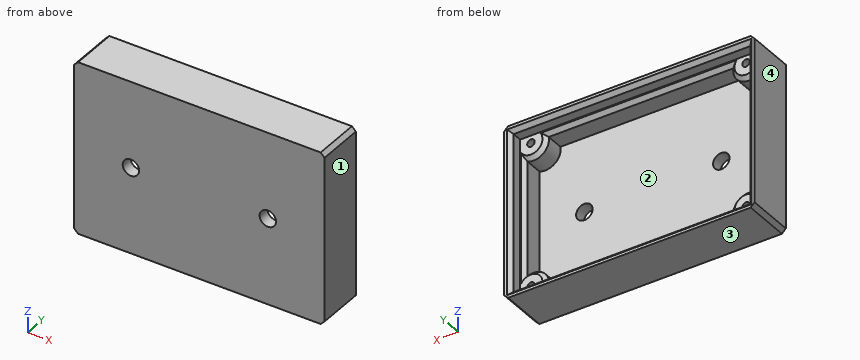
from build123d import *

# Parameters (mm, degrees)
SKETCH1_W           = 64
SKETCH1_H           = 44
BOSS_EXTRUDE1_DEPTH = 12
SKETCH2_W           = 60.5
SKETCH2_H           = 40.5
CUT_EXTRUDE1_DEPTH  = 3.5
SKETCH3_R           = 0.95
CUT_EXTRUDE2_DEPTH  = 6
SHELL1_START        = 3
SHELL1_DEPTH        = 5.5
CHAMFER1_SIZE       = 1
CHAMFER2_SIZE       = 1
CHAMFER3_SIZE       = 1
SKETCH4_R           = 2.1
CUT_EXTRUDE3_DEPTH  = 40.862262856


# Read off the part's stored shape, not the designer's step: Shell1
with BuildPart() as part:
    # Sketch1 → Boss-Extrude1 (new body)
    with BuildSketch(Plane(origin=(0, 0, 0), x_dir=(1, 0, 0), z_dir=(0, 1, 0))):
        Rectangle(SKETCH1_W, SKETCH1_H)
    extrude(amount=BOSS_EXTRUDE1_DEPTH)

    # Sketch2 → Cut-Extrude1 (cut)
    with BuildSketch(Plane(origin=(0, 12, 0), x_dir=(1, 0, 0), z_dir=(0, 1, 0))):
        Rectangle(SKETCH2_W, SKETCH2_H)
    extrude(amount=-CUT_EXTRUDE1_DEPTH, mode=Mode.SUBTRACT)

    # Sketch3 → Cut-Extrude2 (cut)
    with BuildSketch(Plane(origin=(0, 8.5, 0), x_dir=(1, 0, 0), z_dir=(0, 1, 0))):
        with Locations(Location((-27.5, 18.333333333, 0), (0, 0, 270))):
            Circle(SKETCH3_R)
        with Locations(Location((27.5, 18.333333333, 0), (0, 0, 270))):
            Circle(SKETCH3_R)
        with Locations(Location((27.5, -18.333333333, 0), (0, 0, 270))):
            Circle(SKETCH3_R)
        with Locations(Location((-27.5, -18.333333333, 0), (0, 0, 270))):
            Circle(SKETCH3_R)
    extrude(amount=-CUT_EXTRUDE2_DEPTH, mode=Mode.SUBTRACT)

    # Shell1 outline → Shell1 (cut)
    with BuildSketch(Plane(origin=(0, 0, 0), x_dir=(1, 0, 0), z_dir=(0, 1, 0)).offset(SHELL1_START)):
        with BuildLine():
            Line((-23.60666524, -19), (23.60666524, -19))
            ThreePointArc((23.60666524, -19), (25.030327008, -15.250604784), (29, -14.679226055))
            Line((29, -14.679226055), (29, 14.679226055))
            ThreePointArc((29, 14.679226055), (25.030327008, 15.250604784), (23.60666524, 19))
            Line((23.60666524, 19), (-23.60666524, 19))
            ThreePointArc((-23.60666524, 19), (-25.030327008, 15.250604784), (-29, 14.679226055))
            Line((-29, 14.679226055), (-29, -14.679226055))
            ThreePointArc((-29, -14.679226055), (-25.030327008, -15.250604784), (-23.60666524, -19))
        make_face()
    extrude(amount=SHELL1_DEPTH, mode=Mode.SUBTRACT)

    # Chamfer1
    chamfer1_edges = [part.edges().sort_by_distance(p)[0] for p in [
        (30.25, 12, 0),
        (0, 12, -20.25),
        (-30.25, 12, 0),
        (0, 12, 20.25),
    ]]
    chamfer(chamfer1_edges, length=CHAMFER1_SIZE)

    # Chamfer2
    chamfer2_edges = [part.edges().sort_by_distance(p)[0] for p in [
        (0, 8.5, 19),
        (29, 8.5, 0),
        (0, 8.5, -19),
        (-29, 8.5, 0),
        (-25.030327008, 8.5, -15.250604784),
        (25.030327008, 8.5, -15.250604784),
        (25.030327008, 8.5, 15.250604784),
        (-25.030327008, 8.5, 15.250604784),
    ]]
    chamfer(chamfer2_edges, length=CHAMFER2_SIZE)

    # Chamfer3
    chamfer3_edges = [part.edges().sort_by_distance(p)[0] for p in [
        (-32, 6, 22),
        (-32, 6, -22),
        (32, 6, -22),
        (32, 6, 22),
    ]]
    chamfer(chamfer3_edges, length=CHAMFER3_SIZE)

    # Sketch4 → Cut-Extrude3 (cut, through all)
    with BuildSketch(Plane(origin=(0, 3, 0), x_dir=(1, 0, 0), z_dir=(0, 1, 0))):
        with Locations(Location((-17.5, 0, 0), (0, 0, 270))):
            Circle(SKETCH4_R)
        with Locations(Location((17.5, 0, 0), (0, 0, 270))):
            Circle(SKETCH4_R)
    extrude(amount=-CUT_EXTRUDE3_DEPTH, mode=Mode.SUBTRACT)


solid = part.part
Here's how the part is built. I have some questions about the finished solid (model axes, mm). Face numbers are marked on the shaded views. Coordinates: 2 decimals unless noted, no trailing zeros. Order: outer loops, then holes, each group sorted by start corner. A loop starts at its lowest first (then second) coordinate and runs counter-clockwise, first axis right, second up. Notation, with made-up numbers: M -1.75,-19.75 L 30.25,-19.75 A10 cw 30.25,-14.75 Z; hole C 65,-11.75 d7. An arc over 180 degrees is marked long. Answer as CSV lines item,"result". Start each with the question number.
1. I want a section at D-D, the plane x = 27.5. Write out the boundary of the cut face in (y, z), and give its area (3 significant figures).
2. I want a section at B-B, the plane z = 0. Write out the boundary of the cut face in (x, y).
3. For pin 1 (1 mm diameter, centred on x = 25.5, z = 7, fed in from +Y); pin 2 (2 mm diameter, centred on x = -28, z = -18.5, fed in from +Y); pin 3 (0.6 mm diameter, centred on x = -27.5, z = 18.5, fed in from +Y), each with a flat end and sliding along its axis, tell me the tip position at first contact or that it passes through.
4. I want a section at A-A, the plane x = 17.5. Write out the boundary of the cut face in (y, z), and give its area (3 significant figures).
5. I want a section at C-C, the plane x = -13. Write out the boundary of the cut face in (y, z), and give its area (3 significant figures).
6. We'd pull the mould along X, two halves only. Please class the marked faces 1, 2, 3 and 4: released by +X, released by -X, zero draft, split by the parting line, or undercut.
7. I need wall thicknesses on line 1 (X direction, y = 1.9, z = 0); line 2 (Z direction, x = -3, y = 4.25); line 3 (Z direction, x = 21, y = 9.5). Which ranges of each line are inside material? Lowest first, please. Write a range as [from, to].
Recorded:
1,outline,"M 0,-22 L 12,-22 L 12,-21.25 L 11,-20.25 L 8.5,-20.25 L 8.5,-19.28 L 2.5,-19.28 L 2.5,-17.38 L 8.5,-17.38 L 8.5,-15.38 L 7.5,-14.38 L 3,-14.38 L 3,14.38 L 7.5,14.38 L 8.5,15.38 L 8.5,17.38 L 2.5,17.38 L 2.5,19.28 L 8.5,19.28 L 8.5,20.25 L 11,20.25 L 12,21.25 L 12,22 L 0,22 Z"
1,area,"203 mm2"
2,outline,"M -32,0 L -19.6,0 L -19.6,3 L -29,3 L -29,7.5 L -30,8.5 L -30.25,8.5 L -30.25,11 L -31.25,12 L -32,12 Z; M -15.4,0 L 15.4,0 L 15.4,3 L -15.4,3 Z; M 19.6,0 L 32,0 L 32,12 L 31.25,12 L 30.25,11 L 30.25,8.5 L 30,8.5 L 29,7.5 L 29,3 L 19.6,3 Z"
3,pin 1,"stops at y = 3"
3,pin 2,"stops at y = 8.5"
3,pin 3,"stops at y = 2.5"
4,outline,"M 0,-22 L 12,-22 L 12,-21.25 L 11,-20.25 L 8.5,-20.25 L 8.5,-20 L 7.5,-19 L 3,-19 L 3,-2.1 L 0,-2.1 Z; M 0,2.1 L 3,2.1 L 3,19 L 7.5,19 L 8.5,20 L 8.5,20.25 L 11,20.25 L 12,21.25 L 12,22 L 0,22 Z"
4,area,"163 mm2"
5,outline,"M 0,-22 L 12,-22 L 12,-21.25 L 11,-20.25 L 8.5,-20.25 L 8.5,-20 L 7.5,-19 L 3,-19 L 3,19 L 7.5,19 L 8.5,20 L 8.5,20.25 L 11,20.25 L 12,21.25 L 12,22 L 0,22 Z"
5,area,"175 mm2"
6,face 1,"released by +X"
6,face 2,"undercut"
6,face 3,"zero draft"
6,face 4,"released by -X"
7,line 1,"x = [-32, -19.6], [-15.4, 15.4], [19.6, 32]"
7,line 2,"z = [-22, -19], [19, 22]"
7,line 3,"z = [-22, -20.25], [20.25, 22]"
